The model under review builds one solid part; all positions refer to its coordinate system, in mm. A direction names the side the tool comes from. Give positions to 0.01 mm unless a question says otherwise; leave off trailing zeros. Write each loop counter-clockwise with the first axis right and the second up, starting at its lowest first coordinate (ties: lowest second). Pieces come first, ordered by that corner, then holes.
from build123d import *

# Parameters (mm, degrees)
CUT_EXTRUDE2_DEPTH       = 51
CUT_EXTRUDE2_DEPTH_BACK  = 51
BOSS_EXTRUDE3_DEPTH      = 12.5
BOSS_EXTRUDE3_DEPTH_BACK = 12.5
BOSS_EXTRUDE4_DEPTH      = 11
BOSS_EXTRUDE4_DEPTH_BACK = 11
SKETCH4_8_R              = 5
BOSS_EXTRUDE5_DEPTH      = 40
BOSS_EXTRUDE5_DEPTH_BACK = 40


with BuildPart() as part:
    # Sketch1 → Revolve2 (revolve)
    with BuildSketch(Plane.XY):
        with BuildLine():
            ThreePointArc((-50, 95.31782646), (-49.882033293, 95.640395155), (-49.583797747, 95.810754383))
            Line((-49.583797747, 95.810754383), (-25, 99.99))
            Line((-25, 99.99), (0, 99.99))
            Line((0, 99.99), (0, 95.74))
            Line((0, 95.74), (0, 0))
            Line((0, 0), (-50, 0))
            Line((-50, 0), (-50, 73))
            Line((-50, 73), (-48, 73))
            Line((-48, 73), (-48, 76))
            Line((-48, 76), (-50, 76))
            Line((-50, 76), (-50, 80.58))
            Line((-50, 80.58), (-48, 80.58))
            Line((-48, 80.58), (-48, 83.58))
            Line((-48, 83.58), (-50, 83.58))
            Line((-50, 83.58), (-50, 88.16))
            Line((-50, 88.16), (-48, 88.16))
            Line((-48, 88.16), (-48, 91.16))
            Line((-48, 91.16), (-50, 91.16))
            Line((-50, 91.16), (-50, 95.31782646))
        make_face()
    revolve(axis=Axis((0, 95.74, 0), (0, -1, 0)))

    # Sketch2 → Cut-Extrude2 (cut, two sides)
    with BuildSketch(Plane(origin=(0, 0, 0), x_dir=(0, 0, -1), z_dir=(1, 0, 0))) as cut_extrude2_sk:
        with BuildLine():
            Line((30, 0), (30, 30))
            ThreePointArc((30, 30), (38.689431083, 37.119875503), (45.57, 46))
            Line((45.57, 46), (50, 46))
            Line((50, 46), (50, 0))
            Line((50, 0), (30, 0))
        make_face()
        with BuildLine():
            Line((-30, 0), (-30, 30))
            ThreePointArc((-30, 30), (-38.689431083, 37.119875503), (-45.57, 46))
            Line((-45.57, 46), (-50, 46))
            Line((-50, 46), (-50, 0))
            Line((-50, 0), (-30, 0))
        make_face()
    extrude(amount=CUT_EXTRUDE2_DEPTH, mode=Mode.SUBTRACT)
    extrude(cut_extrude2_sk.sketch, amount=-CUT_EXTRUDE2_DEPTH_BACK, mode=Mode.SUBTRACT)

    # Sketch4 → Boss-Extrude3 (add, two sides)
    with BuildSketch(Plane.XY) as boss_extrude3_sk:
        with BuildLine():
            Line((-40, 0), (40, 0))
            ThreePointArc((40, 0), (0, -40), (-40, 0))
        make_face()
        with BuildLine():
            Line((-37.416573868, -2.5), (37.416573868, -2.5))
            ThreePointArc((37.416573868, -2.5), (0, -37.5), (-37.416573868, -2.5))
        make_face(mode=Mode.SUBTRACT)
    extrude(amount=BOSS_EXTRUDE3_DEPTH)
    extrude(boss_extrude3_sk.sketch, amount=-BOSS_EXTRUDE3_DEPTH_BACK)

    # Sketch4<7> → Boss-Extrude4 (add, two sides)
    with BuildSketch(Plane.XY) as boss_extrude4_sk:
        with BuildLine():
            Line((-37.416573868, -2.5), (37.416573868, -2.5))
            ThreePointArc((37.416573868, -2.5), (0, -37.5), (-37.416573868, -2.5))
        make_face()
    extrude(amount=BOSS_EXTRUDE4_DEPTH)
    extrude(boss_extrude4_sk.sketch, amount=-BOSS_EXTRUDE4_DEPTH_BACK)

    # Sketch4<8> → Boss-Extrude5 (add, two sides)
    with BuildSketch(Plane.XY) as boss_extrude5_sk:
        with Locations((-15, 10)):
            Circle(SKETCH4_8_R)
        with Locations((15, 10)):
            Circle(SKETCH4_8_R)
    extrude(amount=BOSS_EXTRUDE5_DEPTH)
    extrude(boss_extrude5_sk.sketch, amount=-BOSS_EXTRUDE5_DEPTH_BACK)


solid = part.part
1) Insertion check: pin 1 (10 mm diameter, centred on y = 44, z = 30, fed in from +X); pin 2 (3 mm diameter, centred on x = 28.5, y = 65.5, fed in from -Z); pin 3 (10 mm diameter, centred on y = 40.5, z = 33, fed in from +X). Each pin has a flat end and moves straight along its axis. Give the tip position at first contact, or say it passes through.
2) The part is to be moulded in two halves that separate along Y. For faces 1 (the flat face through (0, 46, -47)), 2 (the flat face through (1, -16, 11)), 3 (the flat face through (0, 99.99, 0)), 4 (the cylindrical face through (0.56, 37.01, 38.58)), say which applies: +Y half, -Y half, draft (parallel to the pull), parting line (faces both ways), or undercut.
3) Tool access review of faces 5 (the flat face through (15, 10, 40)), 6 (the flat face through (-1, 15, -30)), 7 (the flat face through (-19, 76, -45)): name each direction out of +Z, -Z, +X, -X, +Y, -Y from which nothing blocks a thin tool from reaching the whole face with its end or side.
4) To check wall thickness, follow probe 1 along Z at (x, y) = (-26, 21.5); probe 2 along Y at (x, z) = (9.5, 17); probe 3 along Y at (x, z) = (-14.5, -30.5). State the ranges of each line that lie inside material, in increasing order.
5) Consider section A-A, the plane y = 10. Give the boundary of the cut face in (x, z).
6) Consider section D-D, the plane z = -35.5. State how many separate pieces and enclosed holes the cut face has, then the cut area to 3 significant figures.
7) Consider section C-C, the plane y = -29. Give the boundary of the cut face in (x, z).
Answer block:
1. pin 1: stops at x = 43.3
1. pin 2: stops at z = -42.08
1. pin 3: stops at x = 41.42
2. face 1: -Y half
2. face 2: undercut
2. face 3: +Y half
2. face 4: undercut
3. face 5: +Z, +X, -X, -Y
3. face 6: -Z
3. face 7: none
4. probe 1: z = -30 to 30
4. probe 2: y = 0 to 99.99
4. probe 3: y = 5.03 to 14.97, 30.33 to 98.5
5. outline: (-40, -30) - (-20, -30) - (-20, -40) - (-10, -40) - (-10, -30) - (10, -30) - (10, -40) - (20, -40) - (20, -30) - (40, -30) arc R50 ccw to (40, 30) - (20, 30) - (20, 40) - (10, 40) - (10, 30) - (-10, 30) - (-10, 40) - (-20, 40) - (-20, 30) - (-40, 30) arc R50 ccw to start
6. separate pieces: 3
6. enclosed holes: 0
6. area: 4,560 mm2
7. outline: (-27.55, -12.5) - (-23.77, -12.5) - (-23.77, -11) - (23.77, -11) - (23.77, -12.5) - (27.55, -12.5) - (27.55, 12.5) - (23.77, 12.5) - (23.77, 11) - (-23.77, 11) - (-23.77, 12.5) - (-27.55, 12.5) - close
